For this review, use the dimensioned drawing (mm, ordinates from the lowest corner) and the shaded views. A direction names the side the tool comes from. Give positions to 0.01 mm unless a question says otherwise; leave off trailing zeros. Order: outer loops, then holes, each group sorted by start corner. A loop starts at its lowest first (then second) coordinate and runs counter-clockwise, first axis right, second up. Notation, with made-up numbers: (-32, -34.5) - (24, -34.5) arc R17 ccw to (24, -23.5) - close; hole circle Ø4 at (48.25, 71.25). An arc over 180 degrees is marked (long way). Answer as CSV lines item,"result". Start each with the question number.
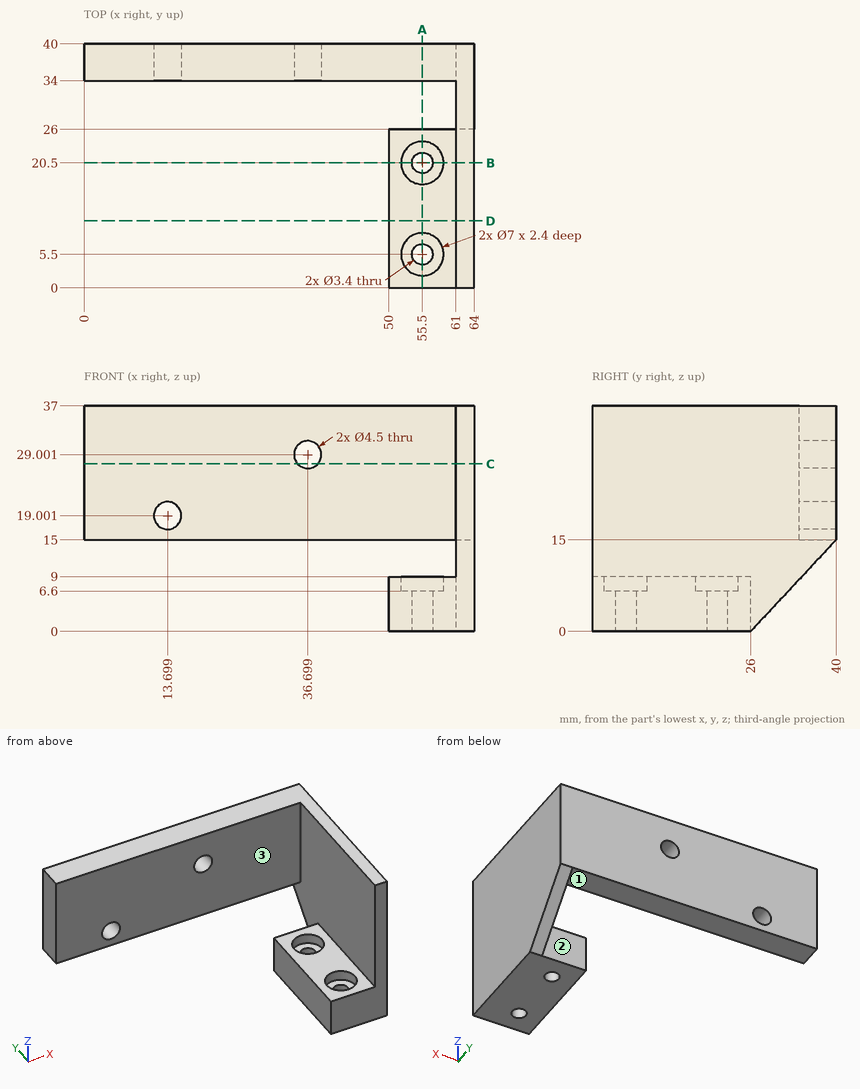
Item 1: Take a section at C-C on z = 27.5. Write out the cut boundary in (x, y) (1 decimal), and give its area (3 significant figures).
Item 2: Clearance check with flat-ended pins moving along their axes: pin 1 (6 mm diameter, centred on y = 17, z = 32.5, fed in from -X); pin 2 (4.5 mm diameter, centred on x = 55.5, y = 20.5, fed in from -Z); pin 3 (6.5 mm diameter, centred on x = 44, z = 25.5, fed in from -Y); pin 4 (10 mm diameter, centred on x = 54.5, z = 5.5, fed in from +Y). State where each tip first meets the part, or that it passes through.
Item 3: Take a section at D-D on y = 11. Write out the cut boundary in (x, z).
Item 4: Take a section at B-B on y = 20.5. Write out the cut boundary in (x, z).
Item 5: Take a section at A-A on x = 55.5. Write out the cut boundary in (y, z).
Item 6: Machinability: for the marked faces 1, 2 and 3, which of the approach directions +Z, -Z, +X, -X, +Y, -Y give a long, thin tool a straight path to every point of the face, cutting with its end or side? Answer none if there is none.
Item 7: For line 1 along Y through (x, z) = (55.5, 8.3); line 2 along Y through (x, z) = (55.5, 3.75); line 3 along X through (y, z) = (12.5, 12), list the stretches that pass through material, from the lowest coordinate up.
Data:
1,outline,"(0, 34) - (35, 34) - (35, 40) - (0, 40) - close; (38.4, 34) - (61, 34) - (61, 0) - (64, 0) - (64, 40) - (38.4, 40) - close"
1,area,"466 mm^2"
2,pin 1,"stops at x = 61"
2,pin 2,"stops at z = 0"
2,pin 3,"stops at y = 34"
2,pin 4,"stops at y = 26"
3,outline,"(50, 0) - (64, 0) - (64, 37) - (61, 37) - (61, 9) - (50, 9) - close"
4,outline,"(50, 0) - (53.8, 0) - (53.8, 6.6) - (52, 6.6) - (52, 9) - (50, 9) - close; (57.2, 0) - (64, 0) - (64, 37) - (61, 37) - (61, 9) - (59, 9) - (59, 6.6) - (57.2, 6.6) - close"
5,outline,"(0, 0) - (3.8, 0) - (3.8, 6.6) - (2, 6.6) - (2, 9) - (0, 9) - close; (7.2, 0) - (18.8, 0) - (18.8, 6.6) - (17, 6.6) - (17, 9) - (9, 9) - (9, 6.6) - (7.2, 6.6) - close; (22.2, 0) - (26, 0) - (26, 9) - (24, 9) - (24, 6.6) - (22.2, 6.6) - close; (34, 15) - (40, 15) - (40, 37) - (34, 37) - close"
6,face 1,"-Z, -X, +Y, -Y"
6,face 2,"+Z, -Z, -X, +Y"
6,face 3,"+Z, -Z, -X, -Y"
7,line 1,"y = 0 to 2, 9 to 17, 24 to 26"
7,line 2,"y = 0 to 3.8, 7.2 to 18.8, 22.2 to 26"
7,line 3,"x = 61 to 64"
